```python
from build123d import *

# Parameters (mm, degrees)
SKETCH1_R           = 4
BOSS_EXTRUDE1_DEPTH = 2
SKETCH2_R           = 2
CUT_EXTRUDE1_DEPTH  = 2


with BuildPart() as part:
    # Sketch1 → Boss-Extrude1 (new body)
    with BuildSketch(Plane.XY):
        Polygon((3.5, 121.5), (12.5, 121.5), (12.5, -121.5), (3.5, -121.5), (0, -121.5), (-12.5, -121.5), (-12.5, -115.487492178), (-12.5, -105.5), (-12.5, 112.5), (-12.5, 121.5), align=None)
        with Locations((0, 109)):
            Circle(SKETCH1_R, mode=Mode.SUBTRACT)
        with Locations(Location((0, -109, 0), (0, 0, 180))):
            Circle(SKETCH1_R, mode=Mode.SUBTRACT)
    extrude(amount=BOSS_EXTRUDE1_DEPTH)

    # Sketch2 → Cut-Extrude1 (cut)
    with BuildSketch(Plane.XY.offset(2)):
        with Locations((1.5, 83.3)):
            Circle(SKETCH2_R)
        with Locations((1.5, 50)):
            Circle(SKETCH2_R)
        with Locations((1.5, 16.7)):
            Circle(SKETCH2_R)
        with Locations((1.5, -16.7)):
            Circle(SKETCH2_R)
        with Locations((1.5, -50)):
            Circle(SKETCH2_R)
        with Locations((1.5, -83.3)):
            Circle(SKETCH2_R)
    extrude(amount=-CUT_EXTRUDE1_DEPTH, mode=Mode.SUBTRACT)


solid = part.part
```
Part model, mm, in its own coordinate system. Coordinates: 2 decimals unless noted, no trailing zeros. Order: outer loops, then holes, each group sorted by start corner. A loop starts at its lowest first (then second) coordinate and runs counter-clockwise, first axis right, second up. Notation, with made-up numbers: (53, 2) -> (102, 2) arc R20 ccw to (102, 11) -> close; hole circle Ø7 at (-38, -36). An arc over 180 degrees is marked (long way). Put each result on its own line as item: value. Start each with the question number.
(1) Band-saw the part on A-A (y = 50). Give the cut face in (x, z).
(2) Pin check, flat tip, straight feed: pin 1 Ø3.5 at (x, y) = (1.5, -83.3) entering from +Z. Stop position of the tip, or through.
(3) Probe line 1 along X through (y, z) = (-109, 0.95). List the from-to ranges inside material, lowest first. Write a range as [from, to].
(4) Mould opens along Y. For faces 1 (the face through (0.521, -112.966, 0.986)), 2 (the face through (0, 2, 0)) say: pulls with the +Y half, pulls with the -Y half, needs draft (parallel to the pull), parting line crosses it, or undercut.
(5) Band-saw the part on B-B (z = 1.5). Count the separate pieces of the cut face and the enclosed holes in it, then the cut area to 3 significant figures.
Determined:
1. outline: (-12.5, 0) -> (-0.5, 0) -> (-0.5, 2) -> (-12.5, 2) -> close; (3.5, 0) -> (12.5, 0) -> (12.5, 2) -> (3.5, 2) -> close
2. pin 1: passes through
3. line 1: x = [-12.5, -4], [4, 12.5]
4. face 1: undercut
4. face 2: needs draft
5. separate pieces: 1
5. enclosed holes: 8
5. area: 5,900 mm²
